from build123d import *

# Parameters (mm, degrees)
SKETCH1_W           = 120
SKETCH1_H           = 180
SKETCH1_R           = 3
BOSS_EXTRUDE1_DEPTH = 10
SKETCH2_W           = 96
SKETCH2_H           = 60
BOSS_EXTRUDE2_DEPTH = 10
SKETCH8_R           = 4
SKETCH8_W           = 2.177957771
SKETCH8_H           = 10
SKETCH8_W_2         = 10
SKETCH8_H_2         = 2.18
CUT_EXTRUDE8_DEPTH  = 231.705439901
SKETCH7_W           = 16.5
SKETCH7_H           = 38
CUT_EXTRUDE7_DEPTH  = 2
SKETCH5_W           = 44
SKETCH5_H           = 44
CUT_EXTRUDE5_DEPTH  = 2


with BuildPart() as part:
    # Sketch1 → Boss-Extrude1 (new body)
    with BuildSketch(Plane(origin=(0, 0, 0), x_dir=(1, 0, 0), z_dir=(0, 1, 0))):
        with Locations((-115, -60)):
            Rectangle(SKETCH1_W, SKETCH1_H)
        with Locations(Location((-163, -138, 0), (0, 0, 270))):
            Circle(SKETCH1_R, mode=Mode.SUBTRACT)
        with Locations(Location((-67, -138, 0), (0, 0, 90))):
            Circle(SKETCH1_R, mode=Mode.SUBTRACT)
        with Locations(Location((-163, 18, 0), (0, 0, 90))):
            Circle(SKETCH1_R, mode=Mode.SUBTRACT)
        with Locations(Location((-67, 18, 0), (0, 0, 270))):
            Circle(SKETCH1_R, mode=Mode.SUBTRACT)
        Polygon((-163, 6), (-163, -126), (-151, -126), (-151, -138), (-79, -138), (-79, -126), (-67, -126), (-67, 6), (-79, 6), (-79, 18), (-151, 18), (-151, 6), align=None, mode=Mode.SUBTRACT)
    extrude(amount=BOSS_EXTRUDE1_DEPTH)

    # Sketch2 → Boss-Extrude2 (add)
    with BuildSketch(Plane(origin=(0, 0, 0), x_dir=(1, 0, 0), z_dir=(0, 1, 0))):
        with Locations((-115, -60)):
            Rectangle(SKETCH2_W, SKETCH2_H)
    extrude(amount=BOSS_EXTRUDE2_DEPTH)

    # Sketch8 → Cut-Extrude8 (cut, through all)
    with BuildSketch(Plane(origin=(0, 10, 0), x_dir=(1, 0, 0), z_dir=(0, 1, 0))):
        with Locations(Location((-169, 6, 0), (0, 0, 270))):
            Circle(SKETCH8_R)
        with Locations(Location((-169, -126.077692428, 0), (0, 0, 90))):
            Circle(SKETCH8_R)
        with Locations(Location((-61, -126.077692428, 0), (0, 0, 270))):
            Circle(SKETCH8_R)
        with Locations(Location((-61, 6, 0), (0, 0, 90))):
            Circle(SKETCH8_R)
        with Locations((-168.898595302, -59.479320644)):
            Rectangle(SKETCH8_W, SKETCH8_H)
        with Locations((-115, 24.434155691)):
            Rectangle(SKETCH8_W_2, SKETCH8_H_2)
        with Locations((-61.101404698, -59.479320644)):
            Rectangle(SKETCH8_W, SKETCH8_H)
        with Locations((-115, -144.434155691)):
            Rectangle(SKETCH8_W_2, SKETCH8_H_2)
    extrude(amount=-CUT_EXTRUDE8_DEPTH, mode=Mode.SUBTRACT)

    # Sketch7 → Cut-Extrude7 (cut)
    with BuildSketch(Plane(origin=(0, 10, 0), x_dir=(1, 0, 0), z_dir=(0, 1, 0))):
        with Locations((-93.25, -52)):
            Rectangle(SKETCH7_W, SKETCH7_H)
    extrude(amount=-CUT_EXTRUDE7_DEPTH, mode=Mode.SUBTRACT)

    # Sketch5 → Cut-Extrude5 (cut)
    with BuildSketch(Plane(origin=(0, 10, 0), x_dir=(1, 0, 0), z_dir=(0, 1, 0))):
        with Locations((-126.5, -55)):
            Rectangle(SKETCH5_W, SKETCH5_H)
    extrude(amount=-CUT_EXTRUDE5_DEPTH, mode=Mode.SUBTRACT)


solid = part.part
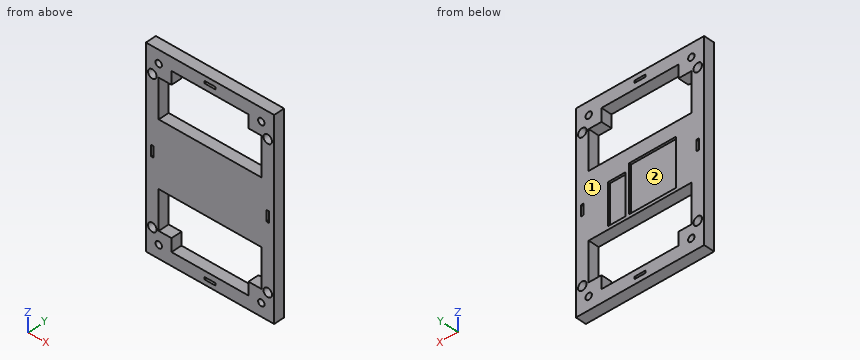
For this review, take the finished solid that the model builds, in its own axes (mm). Face numbers are marked on the shaded views. Round coordinates to 2 decimals unless told otherwise and drop trailing zeros. Loops run counter-clockwise (first coordinate to the right, second up) from the corner with the lowest first, then second, coordinate; pieces in that order, holes last. Notation, with made-up numbers: (-38, 88) - (-28, 88) arc R19 ccw to (-28, 104) - close; hole circle Ø6 at (30, 0). An arc over 180 degrees is marked (long way). Use one line per item in the form item = value.
Item 1: Consider section C-C on y = 1.5. State how many separate pieces and enclosed holes the cut face has, then the cut area to 3 significant figures.
Answers:
separate_pieces = 1
enclosed_holes = 14
area = 12,600 mm^2
Item 2: Consider section A-A on z = 119. Write out the cut boundary in (x, y), then the cut area to 3 significant figures.
Answers:
outline = (-175, 0) - (-163, 0) - (-163, 10) - (-175, 10) - close; (-67, 0) - (-55, 0) - (-55, 10) - (-67, 10) - close
area = 240 mm^2
Item 3: Clearance check with flat-ended pins moving along their axes: P1, Ø3.5, axis at x = -163, z = -18, coming from the +Y side; P2, Ø8, axis at x = -67, z = -18, coming from the +Y side. State where each tip first meets the part, or that it passes through.
Answers:
P1 = through
P2 = 10
Item 4: For line 1 (Z direction, x = -126, y = 3.75); line 2 (Z direction, x = -77.5, y = 0.75); line 3 (Z direction, x = -111, y = 2), list the stretches that pass through material, from the lowest coordinate up.
Answers:
line_1 = -30 to -18, 30 to 90, 138 to 150
line_2 = -30 to -6, 30 to 90, 126 to 150
line_3 = -30 to -25.52, -23.34 to -18, 30 to 90, 138 to 143.34, 145.52 to 150
Item 5: Consider section B-B on x = -142. Write out the cut boundary in (y, z).
Answers:
outline = (0, -30) - (10, -30) - (10, -18) - (0, -18) - close; (0, 30) - (10, 30) - (10, 33) - (8, 33) - (8, 77) - (10, 77) - (10, 90) - (0, 90) - close; (0, 138) - (10, 138) - (10, 150) - (0, 150) - close
Item 6: Mouldability with a two-part tool opening along Z and no side actions: class the marked faces 1 and 2 as +Z half, -Z half, draft (parallel to the pull), parting line (faces both ways), or undercut.
Answers:
face_1 = draft
face_2 = undercut
